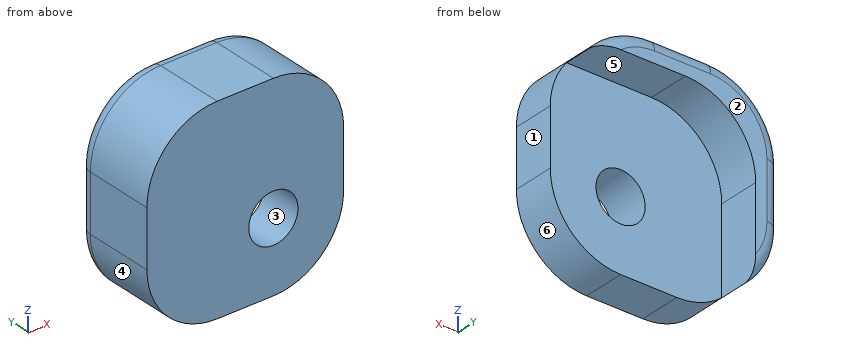
Autodesk Inventor part; units mm, degrees
ref_plane "YZ Plane" through (0, 0, 0) normal (1, 0, 0) x (0, 1, 0)
ref_plane "XZ Plane" through (0, 0, 0) normal (0, 1, 0) x (-1, 0, 0)
ref_plane "XY Plane" through (0, 0, 0) normal (0, 0, 1) x (1, 0, 0)
sketch "Sketch1" plane through (0, 0, 0) normal (0, 1, 0) x (-1, 0, 0)
  line L0 (0, 0) -> (14, 0)
  line L1 (14, 0) -> (14, 14)
  line L2 (14, 14) -> (0, 14)
  line L3 (0, 14) -> (0, 0)
  circle A0 centre (5, 5) radius 1.75
  line L4 (0, 0) -> (12.2, 0)
  line L5 (12.2, 0) -> (12.2, 12.2)
  line L6 (12.2, 12.2) -> (0, 12.2)
  line L7 (0, 12.2) -> (0, 0)
  dimension "d0" = 14
  dimension "d1" = 14
  dimension "d2" = 3.5
  dimension "d3" = 5
  dimension "d4" = 5
  dimension "d5" = 12.2
  dimension "d6" = 12.2
extrude "Extrusion3" add sketch "Sketch1" along normal blind 3 contours L3 L6 L5 L0
extrude "Extrusion4" add sketch "Sketch1" along normal blind 6 contours L5 L6 L3 L2 L1 L0
fillet "Fillet1" radius 5 5 edges at (-14, 3, 0) (-14, 3, 14) (-12.2, 4.5, 12.2) (0, 3, 14) (0, 1.5, 0)
fillet "Fillet2" radius 1 5 edges at (-12.5355, 6, 12.5355) (-7, 6, 14) (-2.8787, 6, 13.5277) (-13.5277, 6, 2.8787) (-14, 6, 7)
properties part number "RxBoardMountFoot"
Source: CAD feature listing. Evaluate the final solid. Frame: model axes, mm. Face numbers are marked on the shaded views. A direction names the side the tool comes from. Give positions to 0.01 mm unless a question says otherwise; leave off trailing zeros. Write each loop counter-clockwise with the first axis right and the second up, starting at its lowest first coordinate (ties: lowest second). Pieces come first, ordered by that corner, then holes. Notation, with made-up numbers: M 7,23 L 16,23 A30 cw 16,61 Z; hole C 30,15 d9. An arc over 180 degrees is marked long. Return JSON: item names as keys, results as strings. Group by question number.
1) Cut plane C-C, the plane z = 8.25. Output: boundary loops of the cut face in (x, y).
2) Pull-direction query (X, two-part tool) for the marked faces 1, 2, 3 and 4; classes: pulls with the +X half, pulls with the -X half, needs draft (parallel to the pull), parting line crosses it, or undercut.
3) Set-up query: the marked faces 5 and 6. Return all of +Z, -Z, +X, -X, +Y, -Y with unobstructed straight access to the full face (end or side cutting, diameter ignored); none if empty.
4) Cut plane B-B, the plane x = -6.5. Output: boundary loops of the cut face in (y, z).
5) Cut plane A-A, the plane y = 2.5. Output: boundary loops of the cut face in (x, z), plus the area to 3 significant figures.
6) Pin query (flat end, axial travel): P1, Ø1.5, axis at y = 4, z = 4, coming from the +X side; P2, Ø3, axis at x = -4, z = 6.5, coming from the +Y side; P3, Ø3.5, axis at x = -5.5, y = 5, coming from the -Z side. Return the tip coordinate at first contact, or that it passes through.
7) Material intervals for line 1 along Z through (x, y) = (-5, 2.1); line 2 along Y through (x, z) = (-9, 9); line 3 along X through (y, z) = (5, 7), sorted ascending. Write a range as [from, to].
Recorded:
{
 "1": {"outline": "M -14,0 L 0,0 L 0,3 L -12.09,3 L -12.09,6 L -13,6 A1 ccw -14,5 Z"},
 "2": {"face 1": "pulls with the +X half", "face 2": "needs draft", "face 3": "undercut", "face 4": "pulls with the -X half"},
 "3": {"face 5": "-Z, +X, +Y", "face 6": "-Z, +X, +Y, -Y"},
 "4": {"outline": "M 0,0 L 3,0 L 3,4.1 L 0,4.1 Z; M 0,5.9 L 3,5.9 L 3,12.2 L 6,12.2 L 6,13 A1 ccw 5,14 L 0,14 Z"},
 "5": {"outline": "M -14,5 A5 ccw -9,0 L -5,0 A5 ccw 0,5 L 0,9 A5 ccw -5,14 L -9,14 A5 ccw -14,9 Z; hole C -5,5 d3.5", "area": "165 mm²"},
 "6": {"P1": "stops at x = -12.2", "P2": "stops at y = 3", "P3": "stops at z = 12.2"},
 "7": {"line 1": "z = [0, 3.25], [6.75, 14]", "line 2": "y = [0, 3]", "line 3": "x = [-14, -12.2]"}
}
